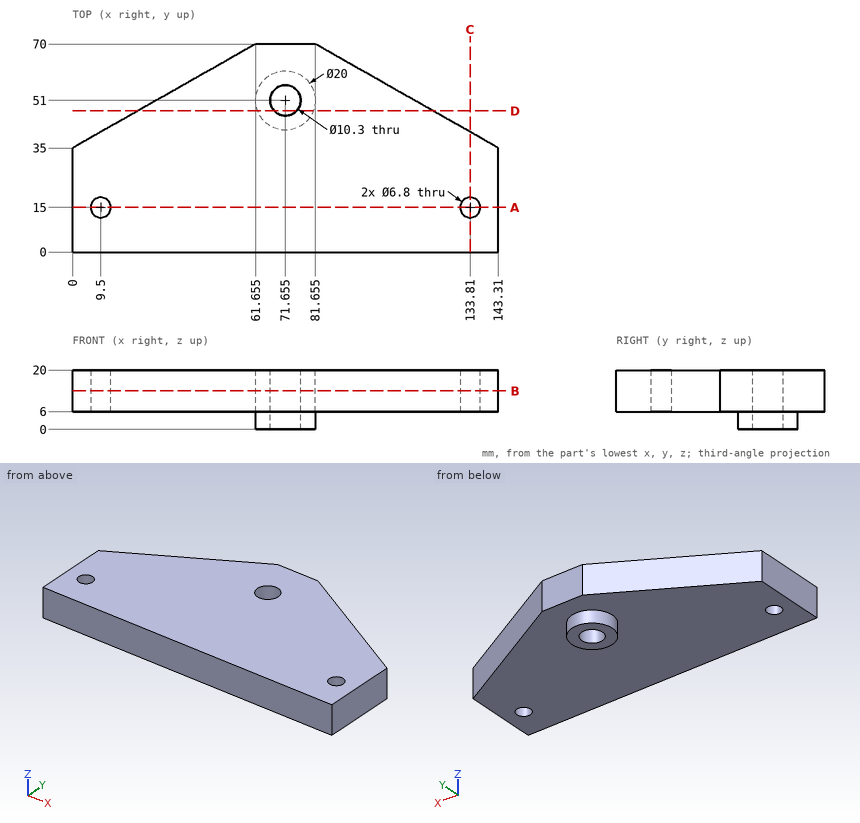
Geometry check sheet. Reference: drawing and pictorial views, mm from the part's lowest x, y, z. Round coordinates to 2 decimals unless told otherwise and drop trailing zeros. Loops run counter-clockwise (first coordinate to the right, second up) from the corner with the lowest first, then second, coordinate; pieces in that order, holes last. Notation, with made-up numbers: (-32.75, 75.5) - (-26.75, 75.5) arc R26 ccw to (-26.75, 90.5) - close; hole circle Ø2 at (-9.75, 14.25). An arc over 180 degrees is marked (long way). Answer in a Markdown table with one row per item. Add a question column.
Q1. Section check D-D on y = 47.5. Enter the section's corners in (x, z), plus the area to 3 significant figures.
Q2. Section check B-B on z = 13. Enter the section's corners in (x, y) (3 decimals).
Q3. Section check C-C on x = 133.81. Enter the section's corners in (y, z).
Q4. Section check A-A on y = 15. Enter the section's corners in (x, z), plus the area to 3 significant figures.
Q5. Gauge pin test, flat ends, axial feed: pin 1 (6 mm diameter, centred on x = 89, z = 5.5, fed in from +Y); pin 2 (8 mm diameter, centred on x = 9.5, y = 15, fed in from -Z); pin 3 (10 mm diameter, centred on x = 36.5, z = 3.5, fed in from +Y). Record the tip position at first contact, or that the pin passes through.
Q6. Material ranges on line 1 (X direction, y = 51, z = 5.5) (3 decimals); line 2 (Z direction, x = 82.5, y = 7); line 3 (Y direction, x = 9.5, z = 12), recorded low to high.
Found:
| question | item | result |
|---|---|---|
| 1 | outline | (22.02, 6) - (62.29, 6) - (62.29, 0) - (67.88, 0) - (67.88, 20) - (22.02, 20) - close; (75.43, 0) - (81.02, 0) - (81.02, 6) - (121.29, 6) - (121.29, 20) - (75.43, 20) - close |
| 1 | area | 1,350 mm² |
| 2 | outline | (0, 0) - (143.31, 0) - (143.31, 35) - (81.655, 70) - (61.655, 70) - (0, 35) - close; hole circle Ø6.8 at (9.5, 15); hole circle Ø10.3 at (71.655, 51); hole circle Ø6.8 at (133.81, 15) |
| 3 | outline | (0, 6) - (11.6, 6) - (11.6, 20) - (0, 20) - close; (18.4, 6) - (40.39, 6) - (40.39, 20) - (18.4, 20) - close |
| 4 | outline | (0, 6) - (6.1, 6) - (6.1, 20) - (0, 20) - close; (12.9, 6) - (130.41, 6) - (130.41, 20) - (12.9, 20) - close; (137.21, 6) - (143.31, 6) - (143.31, 20) - (137.21, 20) - close |
| 4 | area | 1,820 mm² |
| 5 | pin 1 | stops at y = 67.51 |
| 5 | pin 2 | stops at z = 6 |
| 5 | pin 3 | stops at y = 58.18 |
| 6 | line 1 | x = 61.655 to 66.505, 76.805 to 81.655 |
| 6 | line 2 | z = 6 to 20 |
| 6 | line 3 | y = 0 to 11.6, 18.4 to 40.39 |
